Geometry check sheet. Reference: the model listing, model coordinates, mm. A direction names the side the tool comes from. Round coordinates to 2 decimals unless told otherwise and drop trailing zeros. Write each loop counter-clockwise with the first axis right and the second up, starting at its lowest first coordinate (ties: lowest second). Pieces come first, ordered by that corner, then holes. Notation, with made-up numbers: (73, 44) -> (125, 44) arc R20 ccw to (125, 71) -> close; hole circle Ø8 at (-18.5, 25.5). An arc over 180 degrees is marked (long way). Use a Markdown table: item, result.
```python
from build123d import *

# Parameters (mm, degrees)
SKETCH1_W           = 14.6812
SKETCH1_H           = 3.175
BOSS_EXTRUDE1_DEPTH = 2.3749
SKETCH2_W           = 0.5
SKETCH2_H           = 1.5748
BOSS_EXTRUDE2_DEPTH = 2.54
CHAMFER1_SIZE       = 0.381
BOSS_EXTRUDE3_DEPTH = 5.461


with BuildPart() as part:
    # Sketch1 → Boss-Extrude1 (new body, symmetric)
    with BuildSketch(Plane.XY):
        Rectangle(SKETCH1_W, SKETCH1_H)
    extrude(amount=BOSS_EXTRUDE1_DEPTH, both=True)

    # Sketch2 → Boss-Extrude2 (add)
    with BuildSketch(Plane.XZ.offset(1.5875)):
        with Locations((-5.3122, 0)):
            Rectangle(SKETCH2_W, SKETCH2_H)
        with Locations((-2.4852, 0)):
            Rectangle(SKETCH2_W, SKETCH2_H)
        with Locations((2.4852, 0)):
            Rectangle(SKETCH2_W, SKETCH2_H)
        with Locations((5.3122, 0)):
            Rectangle(SKETCH2_W, SKETCH2_H)
    extrude(amount=BOSS_EXTRUDE2_DEPTH)

    # Chamfer1
    chamfer1_edges = [part.edges().sort_by_distance(p)[0] for p in [
        (-5.3122, -4.1275, -0.7874),
        (-5.3122, -4.1275, 0.7874),
        (-2.4852, -4.1275, -0.7874),
        (-2.4852, -4.1275, 0.7874),
        (2.4852, -4.1275, 0.7874),
        (2.4852, -4.1275, -0.7874),
        (5.3122, -4.1275, 0.7874),
        (5.3122, -4.1275, -0.7874),
    ]]
    chamfer(chamfer1_edges, length=CHAMFER1_SIZE)

    # Sketch3 → Boss-Extrude3 (add)
    with BuildSketch(Plane(origin=(0, 1.5875, 0), x_dir=(1, 0, 0), z_dir=(0, 1, 0))):
        Polygon((-5.3082, 0.8763), (-2.4892, 0.8763), (-2.4892, -0.1524), (-3.5812, -0.1524), (-3.5812, -0.4064), (-2.2352, -0.4064), (-2.2352, 1.1303), (-5.5622, 1.1303), (-5.5622, -0.4064), (-4.2162, -0.4064), (-4.2162, -0.1524), (-5.3082, -0.1524), align=None)
        Polygon((5.5622, 1.1303), (5.5622, -0.4064), (4.2162, -0.4064), (4.2162, -0.1524), (5.3082, -0.1524), (5.3082, 0.8763), (2.4892, 0.8763), (2.4892, -0.1524), (3.5812, -0.1524), (3.5812, -0.4064), (2.2352, -0.4064), (2.2352, 1.1303), align=None)
    extrude(amount=BOSS_EXTRUDE3_DEPTH)


solid = part.part
```
(1) Thickness scan on line 1 (X direction, y = -2, z = -0.05); line 2 (Z direction, x = -3, y = 5.75); line 3 (X direction, y = 6, z = 0.3). Record the ranges inside material, lowest first.
A:
| item | result |
|---|---|
| line 1 | x = -5.56 to -5.06, -2.74 to -2.24, 2.24 to 2.74, 5.06 to 5.56 |
| line 2 | z = -1.13 to -0.88, 0.15 to 0.41 |
| line 3 | x = -5.56 to -4.22, -3.58 to -2.24, 2.24 to 3.58, 4.22 to 5.56 |
(2) Section check C-C on x = -4. Record the cut outline in (y, z).
A:
| item | result |
|---|---|
| outline | (-1.59, -2.37) -> (1.59, -2.37) -> (1.59, -1.13) -> (7.05, -1.13) -> (7.05, -0.88) -> (1.59, -0.88) -> (1.59, 2.37) -> (-1.59, 2.37) -> close |
(3) Section check B-B on y = 4.5. Record the cut outline in (x, z), plus the area to 3 significant figures.
A:
| item | result |
|---|---|
| outline | (-5.56, -1.13) -> (-2.24, -1.13) -> (-2.24, 0.41) -> (-3.58, 0.41) -> (-3.58, 0.15) -> (-2.49, 0.15) -> (-2.49, -0.88) -> (-5.31, -0.88) -> (-5.31, 0.15) -> (-4.22, 0.15) -> (-4.22, 0.41) -> (-5.56, 0.41) -> close; (2.24, -1.13) -> (5.56, -1.13) -> (5.56, 0.41) -> (4.22, 0.41) -> (4.22, 0.15) -> (5.31, 0.15) -> (5.31, -0.88) -> (2.49, -0.88) -> (2.49, 0.15) -> (3.58, 0.15) -> (3.58, 0.41) -> (2.24, 0.41) -> close |
| area | 4.10 mm2 |
(4) Gauge pin test, flat ends, axial feed: pin 1 Ø1.1 at (x, y) = (-4.5, 3) entering from +Z; pin 2 Ø1.7 at (y, z) = (5, -0.5) entering from +X; pin 3 Ø1 at (x, y) = (-4.5, 4.5) entering from -Z. Record the tip position at first contact, or that the pin passes through.
A:
| item | result |
|---|---|
| pin 1 | stops at z = 0.41 |
| pin 2 | stops at x = 5.56 |
| pin 3 | stops at z = -1.13 |
(5) Section check D-D on z = -2.1. Record the cut outline in (x, y).
A:
| item | result |
|---|---|
| outline | (-7.34, -1.59) -> (7.34, -1.59) -> (7.34, 1.59) -> (-7.34, 1.59) -> close |
(6) Access from +Z, -Z, +X, -X, +Y, -Y to the whole of each face (thin tool, end or side, straight path). Record for faces 1 (the face through (-5.562, 4, 0)), 2 (the face through (-3, 4, 0.152)), 3 (the face through (-2.235, -3, 0)).
A:
| item | result |
|---|---|
| face 1 | +Z, -Z, -X, +Y |
| face 2 | +Y |
| face 3 | +Z, -Z, -Y |
(7) Section check A-A on y = -3. Record the cut outline in (x, z), plus the area to 3 significant figures.
A:
| item | result |
|---|---|
| outline | (-5.56, -0.79) -> (-5.06, -0.79) -> (-5.06, 0.79) -> (-5.56, 0.79) -> close; (-2.74, -0.79) -> (-2.24, -0.79) -> (-2.24, 0.79) -> (-2.74, 0.79) -> close; (2.24, -0.79) -> (2.74, -0.79) -> (2.74, 0.79) -> (2.24, 0.79) -> close; (5.06, -0.79) -> (5.56, -0.79) -> (5.56, 0.79) -> (5.06, 0.79) -> close |
| area | 3.15 mm2 |
(8) Release check for a two-part mould opening along X. For faces 4 (the face through (3, 4, 0.152)), 5 (the face through (3, 4, 0.406)), 6 (the face through (2.235, 4, 0)), 7 (the face through (-5.562, -3, 0)) record: +X half, -X half, draft (parallel to the pull), parting line (faces both ways), or undercut.
A:
| item | result |
|---|---|
| face 4 | undercut |
| face 5 | draft |
| face 6 | undercut |
| face 7 | -X half |
